```python
from build123d import *

# Parameters (mm, degrees)
SKETCH1_W           = 220
SKETCH1_H           = 120
BOSS_EXTRUDE1_DEPTH = 10
CUT_EXTRUDE1_REACH  = 127.698
SKETCH2_W           = 20.632503002
SKETCH2_H           = 54.730004003
CUT_EXTRUDE2_REACH  = 127.698
SKETCH3_R           = 10


with BuildPart() as part:
    # Sketch1 → Boss-Extrude1 (new body)
    with BuildSketch(Plane(origin=(0, 0, 0), x_dir=(1, 0, 0), z_dir=(0, 1, 0))):
        Rectangle(SKETCH1_W, SKETCH1_H)
    extrude(amount=-BOSS_EXTRUDE1_DEPTH)

    # Sketch2 → Cut-Extrude1 (cut, up to next)
    with BuildSketch(Plane(origin=(0, 0, 0), x_dir=(1, 0, 0), z_dir=(0, 1, 0)), mode=Mode.PRIVATE) as cut_extrude1_sk1:
        with Locations((-99.683748499, 32.634997999)):
            Rectangle(SKETCH2_W, SKETCH2_H)
    cut_extrude1_tool1 = extrude(cut_extrude1_sk1.sketch, amount=-CUT_EXTRUDE1_REACH, mode=Mode.PRIVATE) & part.part
    add(cut_extrude1_tool1.solids().sort_by_distance((-99.683748, 0, -32.634998))[0], mode=Mode.SUBTRACT)

    # Sketch3 → Cut-Extrude2 (cut, up to next)
    with BuildSketch(Plane(origin=(0, 0, 0), x_dir=(1, 0, 0), z_dir=(0, 1, 0)), mode=Mode.PRIVATE) as cut_extrude2_sk1:
        with Locations(Location((97.816251501, -47, 0), (0, 0, 270))):
            Circle(SKETCH3_R)
    cut_extrude2_tool1 = extrude(cut_extrude2_sk1.sketch, amount=-CUT_EXTRUDE2_REACH, mode=Mode.PRIVATE) & part.part
    # Sketch3 → Cut-Extrude2 (cut, up to next)
    with BuildSketch(Plane(origin=(0, 0, 0), x_dir=(1, 0, 0), z_dir=(0, 1, 0)), mode=Mode.PRIVATE) as cut_extrude2_sk2:
        with Locations(Location((-77.183748499, -47, 0), (0, 0, 270))):
            Circle(SKETCH3_R)
    cut_extrude2_tool2 = extrude(cut_extrude2_sk2.sketch, amount=-CUT_EXTRUDE2_REACH, mode=Mode.PRIVATE) & part.part
    # Sketch3 → Cut-Extrude2 (cut, up to next)
    with BuildSketch(Plane(origin=(0, 0, 0), x_dir=(1, 0, 0), z_dir=(0, 1, 0)), mode=Mode.PRIVATE) as cut_extrude2_sk3:
        with Locations(Location((-70, -14.72, 0), (0, 0, 270))):
            Circle(SKETCH3_R)
    cut_extrude2_tool3 = extrude(cut_extrude2_sk3.sketch, amount=-CUT_EXTRUDE2_REACH, mode=Mode.PRIVATE) & part.part
    # Sketch3 → Cut-Extrude2 (cut, up to next)
    with BuildSketch(Plane(origin=(0, 0, 0), x_dir=(1, 0, 0), z_dir=(0, 1, 0)), mode=Mode.PRIVATE) as cut_extrude2_sk4:
        with Locations(Location((-50, 0.28, 0), (0, 0, 270))):
            Circle(SKETCH3_R)
    cut_extrude2_tool4 = extrude(cut_extrude2_sk4.sketch, amount=-CUT_EXTRUDE2_REACH, mode=Mode.PRIVATE) & part.part
    # Sketch3 → Cut-Extrude2 (cut, up to next)
    with BuildSketch(Plane(origin=(0, 0, 0), x_dir=(1, 0, 0), z_dir=(0, 1, 0)), mode=Mode.PRIVATE) as cut_extrude2_sk5:
        with Locations(Location((30, -7.72, 0), (0, 0, 270))):
            Circle(SKETCH3_R)
    cut_extrude2_tool5 = extrude(cut_extrude2_sk5.sketch, amount=-CUT_EXTRUDE2_REACH, mode=Mode.PRIVATE) & part.part
    # Sketch3 → Cut-Extrude2 (cut, up to next)
    with BuildSketch(Plane(origin=(0, 0, 0), x_dir=(1, 0, 0), z_dir=(0, 1, 0)), mode=Mode.PRIVATE) as cut_extrude2_sk6:
        with Locations(Location((62.816251501, -7.72, 0), (0, 0, 270))):
            Circle(SKETCH3_R)
    cut_extrude2_tool6 = extrude(cut_extrude2_sk6.sketch, amount=-CUT_EXTRUDE2_REACH, mode=Mode.PRIVATE) & part.part
    # Sketch3 → Cut-Extrude2 (cut, up to next)
    with BuildSketch(Plane(origin=(0, 0, 0), x_dir=(1, 0, 0), z_dir=(0, 1, 0)), mode=Mode.PRIVATE) as cut_extrude2_sk7:
        with Locations(Location((55.316251501, 20, 0), (0, 0, 270))):
            Circle(SKETCH3_R)
    cut_extrude2_tool7 = extrude(cut_extrude2_sk7.sketch, amount=-CUT_EXTRUDE2_REACH, mode=Mode.PRIVATE) & part.part
    # Sketch3 → Cut-Extrude2 (cut, up to next)
    with BuildSketch(Plane(origin=(0, 0, 0), x_dir=(1, 0, 0), z_dir=(0, 1, 0)), mode=Mode.PRIVATE) as cut_extrude2_sk8:
        with Locations(Location((97.816251501, 47, 0), (0, 0, 270))):
            Circle(SKETCH3_R)
    cut_extrude2_tool8 = extrude(cut_extrude2_sk8.sketch, amount=-CUT_EXTRUDE2_REACH, mode=Mode.PRIVATE) & part.part
    # Sketch3 → Cut-Extrude2 (cut, up to next)
    with BuildSketch(Plane(origin=(0, 0, 0), x_dir=(1, 0, 0), z_dir=(0, 1, 0)), mode=Mode.PRIVATE) as cut_extrude2_sk9:
        with Locations(Location((-34.683748499, 20, 0), (0, 0, 270))):
            Circle(SKETCH3_R)
    cut_extrude2_tool9 = extrude(cut_extrude2_sk9.sketch, amount=-CUT_EXTRUDE2_REACH, mode=Mode.PRIVATE) & part.part
    # Sketch3 → Cut-Extrude2 (cut, up to next)
    with BuildSketch(Plane(origin=(0, 0, 0), x_dir=(1, 0, 0), z_dir=(0, 1, 0)), mode=Mode.PRIVATE) as cut_extrude2_sk10:
        with Locations(Location((-77.183748499, 47, 0), (0, 0, 270))):
            Circle(SKETCH3_R)
    cut_extrude2_tool10 = extrude(cut_extrude2_sk10.sketch, amount=-CUT_EXTRUDE2_REACH, mode=Mode.PRIVATE) & part.part
    add(cut_extrude2_tool1.solids().sort_by_distance((97.816252, 0, 47))[0], mode=Mode.SUBTRACT)
    add(cut_extrude2_tool2.solids().sort_by_distance((-77.183748, 0, 47))[0], mode=Mode.SUBTRACT)
    add(cut_extrude2_tool3.solids().sort_by_distance((-70, 0, 14.72))[0], mode=Mode.SUBTRACT)
    add(cut_extrude2_tool4.solids().sort_by_distance((-50, 0, -0.28))[0], mode=Mode.SUBTRACT)
    add(cut_extrude2_tool5.solids().sort_by_distance((30, 0, 7.72))[0], mode=Mode.SUBTRACT)
    add(cut_extrude2_tool6.solids().sort_by_distance((62.816252, 0, 7.72))[0], mode=Mode.SUBTRACT)
    add(cut_extrude2_tool7.solids().sort_by_distance((55.316252, 0, -20))[0], mode=Mode.SUBTRACT)
    add(cut_extrude2_tool8.solids().sort_by_distance((97.816252, 0, -47))[0], mode=Mode.SUBTRACT)
    add(cut_extrude2_tool9.solids().sort_by_distance((-34.683748, 0, -20))[0], mode=Mode.SUBTRACT)
    add(cut_extrude2_tool10.solids().sort_by_distance((-77.183748, 0, -47))[0], mode=Mode.SUBTRACT)


solid = part.part
```
CAD build for the part. Positions are in the model's coordinates, mm. A direction names the side the tool comes from. Round coordinates to 2 decimals unless told otherwise and drop trailing zeros. Order: outer loops, then holes, each group sorted by start corner. A loop starts at its lowest first (then second) coordinate and runs counter-clockwise, first axis right, second up.
Q1. Slice it at D-D (y = -2). State how many separate pieces and enclosed holes the cut face has, and give its area (3 significant figures).
Q2. Slice it at B-B (z = 2). Write the cut outline in (x, y), and give its area (3 significant figures).
Q3. Which spindle directions (+Z, -Z, +X, -X, +Y, -Y) get a long thin tool onto all of the face, cutting with end or side? Do faces 4 (the cylindrical face through (21.128, -4.93, 12.334)), 5 (the flat face through (-100, -5, -5.27)). Say none if no direction does.
Q4. Two-plate mould, pull along Z, no slides. Class faces 1 (the flat face through (-2, -5, 60)), 2 (the flat face through (-2, -10, -1)), 3 (the cylindrical face through (-67.27, -4.93, 45.7)): pulls with the +Z half, pulls with the -Z half, needs draft (parallel to the pull), parting line crosses it, or undercut.
Q5. Slice it at C-C (x = -70). Write the cut outline in (y, z), and give its area (3 significant figures).
Q6. Wall check: L1, parallel to X at y = -6.25, z = -47; L2, parallel to X at y = -5, z = 47; L3, parallel to X at y = -6.75, z = 12.5. Give the ranges that are in metal, low to high.
Q7. Drop flat-ended pins along their axis: pin 1 (16 mm diameter, centred on x = 55.32, z = -20, fed in from -Y); pin 2 (3 mm diameter, centred on x = -102.5, y = -5, fed in from -Z). Give the stop position or say it passes through.
Q8. Slice it at A-A (z = -47). Write the cut outline in (x, y), and give its area (3 significant figures).
Results below:
1. separate pieces: 1
1. enclosed holes: 10
1. area: 22,100 mm2
2. outline: (-110, -10) - (-59.74, -10) - (-59.74, 0) - (-110, 0) - close; (-40.26, -10) - (21.8, -10) - (21.8, 0) - (-40.26, 0) - close; (38.2, -10) - (54.61, -10) - (54.61, 0) - (38.2, 0) - close; (71.02, -10) - (110, -10) - (110, 0) - (71.02, 0) - close
2. area: 1,680 mm2
3. face 4: +Y, -Y
3. face 5: -Z, -X, +Y, -Y
4. face 1: pulls with the +Z half
4. face 2: needs draft
4. face 3: undercut
5. outline: (-10, -60) - (0, -60) - (0, -53.96) - (-10, -53.96) - close; (-10, -40.04) - (0, -40.04) - (0, 4.72) - (-10, 4.72) - close; (-10, 24.72) - (0, 24.72) - (0, 40.04) - (-10, 40.04) - close; (-10, 53.96) - (0, 53.96) - (0, 60) - (-10, 60) - close
5. area: 722 mm2
6. L1: x = -89.37 to -87.18, -67.18 to 87.82, 107.82 to 110
6. L2: x = -110 to -87.18, -67.18 to 87.82, 107.82 to 110
6. L3: x = -110 to -79.75, -60.25 to 21.22, 38.78 to 54.03, 71.6 to 110
7. pin 1: passes through
7. pin 2: stops at z = -5.27
8. outline: (-89.37, -10) - (-87.18, -10) - (-87.18, 0) - (-89.37, 0) - close; (-67.18, -10) - (87.82, -10) - (87.82, 0) - (-67.18, 0) - close; (107.82, -10) - (110, -10) - (110, 0) - (107.82, 0) - close
8. area: 1,590 mm2
